The model under review builds one solid part; all positions refer to its coordinate system, in mm. A direction names the side the tool comes from. Round coordinates to 2 decimals unless told otherwise and drop trailing zeros. Loops run counter-clockwise (first coordinate to the right, second up) from the corner with the lowest first, then second, coordinate; pieces in that order, holes last. Notation, with made-up numbers: M 3,71 L 37,71 A27 cw 37,99 Z; hole C 3,-11 d10. An arc over 180 degrees is marked long. One line per question, with ' | ' between items.
from build123d import *

# Parameters (mm, degrees)
BOSS_EXTRUDE1_DEPTH = 5
SKETCH2_R           = 2.1
CUT_EXTRUDE1_DEPTH  = 10
SKETCH3_R           = 10
BOSS_EXTRUDE2_DEPTH = 1
SKETCH4_R           = 2.75
BOSS_EXTRUDE3_DEPTH = 5
SKETCH5_W           = 50
SKETCH5_H           = 30
SKETCH5_W_2         = 34
SKETCH5_H_2         = 14
CUT_EXTRUDE2_DEPTH  = 52.14684741
CUT_EXTRUDE3_START  = -1
CUT_EXTRUDE3_DEPTH  = 1
CUT_EXTRUDE4_START  = -1
CUT_EXTRUDE4_DEPTH  = 1
CHAMFER1_SIZE       = 3
CHAMFER2_SIZE       = 3
SKETCH8_W           = 10.980685111
SKETCH8_H           = 18.946061275
CUT_EXTRUDE5_DEPTH  = 51.645829048
BOSS_EXTRUDE4_DEPTH = 1


with BuildPart() as part:
    # Sketch1 → Boss-Extrude1 (new, symmetric)
    with BuildSketch(Plane.XY):
        Polygon((15, 5), (15, 0), (0, 0), (0, 19), (15, 19), (15, 14), (20, 14), (20, 24), (-10, 24), (-10, -5), (20, -5), (20, 5), align=None)
    extrude(amount=BOSS_EXTRUDE1_DEPTH, both=True)

    # Sketch2 → Cut-Extrude1 (cut)
    with BuildSketch(Plane.ZY.offset(10)):
        with Locations(Location((0, 9.5, 0), (0, 0, 270))):
            Circle(SKETCH2_R)
    extrude(amount=-CUT_EXTRUDE1_DEPTH, mode=Mode.SUBTRACT)

    # Sketch3 → Boss-Extrude2 (add)
    with BuildSketch(Plane(origin=(0, 24, 0), x_dir=(1, 0, 0), z_dir=(0, 1, 0))):
        with Locations(Location((0, 0, 0), (0, 0, 180))):
            Circle(SKETCH3_R)
    extrude(amount=BOSS_EXTRUDE2_DEPTH)

    # Sketch4 → Boss-Extrude3 (add)
    with BuildSketch(Plane(origin=(0, 0, 0), x_dir=(0.866025403784438, 0, 0.500000000000001), z_dir=(-0.500000000000001, 0, 0.866025403784438))):
        with BuildLine():
            Line((10, 25), (-10, 25))
            Line((-10, 25), (-4.615384615, 37.923076923))
            ThreePointArc((-4.615384615, 37.923076923), (0, 41), (4.615384615, 37.923076923))
            Line((4.615384615, 37.923076923), (10, 25))
        make_face()
        with Locations((0, 36)):
            Circle(SKETCH4_R, mode=Mode.SUBTRACT)
    extrude(amount=BOSS_EXTRUDE3_DEPTH)

    # Sketch5 → Cut-Extrude2 (cut, through all)
    with BuildSketch(Plane.XZ.offset(5)):
        with Locations((5, 0)):
            Rectangle(SKETCH5_W, SKETCH5_H)
        with Locations((5, 0)):
            Rectangle(SKETCH5_W_2, SKETCH5_H_2, mode=Mode.SUBTRACT)
    extrude(amount=-CUT_EXTRUDE2_DEPTH, mode=Mode.SUBTRACT)

    # Sketch6 → Cut-Extrude3 (cut)
    with BuildSketch(Plane(origin=(0, 25, 0), x_dir=(1, 0, 0), z_dir=(0, 1, 0)).offset(CUT_EXTRUDE3_START)):
        with BuildLine():
            Line((7.141428429, 7), (-7.141428429, 7))
            ThreePointArc((-7.141428429, 7), (-7.963874195, 6.047868038), (-8.660254038, 5))
            Line((-8.660254038, 5), (8.660254038, -5))
            ThreePointArc((8.660254038, -5), (9.920851384, 1.255670262), (7.141428429, 7))
        make_face()
    extrude(amount=CUT_EXTRUDE3_DEPTH, mode=Mode.SUBTRACT)

    # Sketch7 → Cut-Extrude4 (cut)
    with BuildSketch(Plane(origin=(0, 25, 0), x_dir=(1, 0, 0), z_dir=(0, 1, 0)).offset(CUT_EXTRUDE4_START)):
        with BuildLine():
            Line((-7.141428429, -7), (2.124355653, -7))
            Line((2.124355653, -7), (-10, 0))
            ThreePointArc((-10, 0), (-9.257815193, -3.780589618), (-7.141428429, -7))
        make_face()
    extrude(amount=CUT_EXTRUDE4_DEPTH, mode=Mode.SUBTRACT)

    # Chamfer1
    # the kernel refuses this chamfer: 3 mm, written as the material it adds along each edge
    with BuildSketch(Plane(origin=(5.341682432, 24, 8.857524482), x_dir=(0.013747938305293134, 0.9996219169112968, -0.023812127644090214), z_dir=(-0.8660254037844382, 0, -0.500000000000001))) as chamfer1_piece_1_section:
        Polygon((CHAMFER1_SIZE * 0.999621916911, -CHAMFER1_SIZE * 0.0274958766106), (-CHAMFER1_SIZE * 0.0274958766106, -CHAMFER1_SIZE * 0.999621916911), (0, 0), align=None)
    chamfer1_piece_1 = extrude(amount=25.430097928, mode=Mode.PRIVATE)
    chamfer1_piece_1 = split(chamfer1_piece_1, bisect_by=Plane(origin=(-10, 25.699033003, 2.85935222), z_dir=(1, 0, 0)), keep=Keep.TOP, mode=Mode.PRIVATE)
    chamfer1_piece_1 = split(chamfer1_piece_1, bisect_by=Plane(origin=(-6.251324666, 25.699033003, 5), z_dir=(0, 0, -1)), keep=Keep.TOP, mode=Mode.PRIVATE)
    add(chamfer1_piece_1)
    with BuildSketch(Plane(origin=(5.341682432, 24, 8.857524482), x_dir=(0.013747938305293134, 0.9996219169112968, -0.023812127644090214), z_dir=(-0.8660254037844382, 0, -0.500000000000001))) as chamfer1_piece_2_section:
        Polygon((CHAMFER1_SIZE * 0.999621916911, -CHAMFER1_SIZE * 0.0274958766106), (-CHAMFER1_SIZE * 0.0274958766106, -CHAMFER1_SIZE * 0.999621916911), (0, 0), align=None)
    chamfer1_piece_2 = extrude(amount=25.430097928, mode=Mode.PRIVATE)
    chamfer1_piece_2 = split(chamfer1_piece_2, bisect_by=Plane(origin=(-10.676225886, 25, 0.518721071), z_dir=(0, 1, 0)), keep=Keep.TOP, mode=Mode.PRIVATE)
    chamfer1_piece_2 = split(chamfer1_piece_2, bisect_by=Plane(origin=(-11.252418357, 25.835555068, 0.186056192), z_dir=(0.7994080650317889, -0.38461538461538497, 0.46153846153846245)), keep=Keep.TOP, mode=Mode.PRIVATE)
    chamfer1_piece_2 = split(chamfer1_piece_2, bisect_by=Plane(origin=(-10.676225886, 25.558334336, 5), z_dir=(0, 0, -1)), keep=Keep.TOP, mode=Mode.PRIVATE)
    add(chamfer1_piece_2)

    # Chamfer2
    # the kernel refuses this chamfer: 3 mm, written as the material it adds along each edge
    with BuildSketch(Plane(origin=(16.375303002, 24, 5), x_dir=(0, -0.9996219169112968, -0.02749587661058648), z_dir=(-1, 0, 0))) as chamfer2_piece_1_section:
        Polygon((CHAMFER2_SIZE * 0.999621916911, CHAMFER2_SIZE * 0.0274958766106), (-CHAMFER2_SIZE * 0.0274958766106, CHAMFER2_SIZE * 0.999621916911), (0, 0), align=None)
    chamfer2_piece_1 = extrude(amount=25.430097928, mode=Mode.PRIVATE)
    chamfer2_piece_1 = chamfer2_piece_1 & Plane(origin=(0, 22.869371877, 0), x_dir=(-1, 0, 0), z_dir=(0, -1, 0)) * Cylinder(10, 63, mode=Mode.PRIVATE)
    chamfer2_piece_1 = split(chamfer2_piece_1, bisect_by=Plane(origin=(4.051544609, 22.869371877, 7), z_dir=(0, 0, -1)), keep=Keep.TOP, mode=Mode.PRIVATE)
    chamfer2_piece_1 = split(chamfer2_piece_1, bisect_by=Plane(origin=(3.023607395, 22.869371877, 7.519183235), z_dir=(0.500000000000001, 0, -0.8660254037844382)), keep=Keep.TOP, mode=Mode.PRIVATE)
    add(chamfer2_piece_1)

    # Sketch8 → Cut-Extrude5 (cut, through all)
    with BuildSketch(Plane.XZ.offset(5)):
        with Locations((-15.490342555, -3.686972965)):
            Rectangle(SKETCH8_W, SKETCH8_H)
    extrude(amount=-CUT_EXTRUDE5_DEPTH, mode=Mode.SUBTRACT)

    # Sketch9 → Boss-Extrude4 (add)
    with BuildSketch(Plane(origin=(0, 24, 0), x_dir=(1, 0, 0), z_dir=(0, 1, 0))):
        with BuildLine():
            Line((-8.660254038, 5), (-10, 5))
            Line((-10, 5), (-10, 0))
            ThreePointArc((-10, 0), (-9.659258263, 2.588190451), (-8.660254038, 5))
        make_face()
    extrude(amount=BOSS_EXTRUDE4_DEPTH)


solid = part.part
1) Add section B-B on z = -3.75. State the section outline as (x, y) points, then the cut area to 3 significant figures.
Output values:
outline: M -10,-5 L 20,-5 L 20,5 L 15,5 L 15,0 L 0,0 L 0,19 L 15,19 L 15,14 L 20,14 L 20,24 L -6.5,24 L -6.5,31 L -9.38,25 L -10,25 Z | area: 552 mm²
2) Add section D-D on y = 19.5. State the section outline as (x, z) points.
Output values:
outline: M -10,-5 L 20,-5 L 20,5 L -10,5 Z
3) For line 1 (Z direction, x = -6.25, y = 9.5); line 2 (Y direction, x = 13, z = 1); line 3 (X direction, y = 4.5, z = 0.75), list the stretches that pass through material, from the lowest coordinate up.
Output values:
line 1: z = -5 to -2.1, 2.1 to 5 | line 2: y = -5 to 0, 19 to 24 | line 3: x = -10 to 0, 15 to 20
4) Insertion check: P1, Ø2, axis at x = 1.5, y = 25.5, coming from the -Z side; P2, Ø5, axis at x = 1, y = 32.5, coming from the -Z side; P3, Ø0.7, axis at x = -9, z = -4, coming from the +Y side; P4, Ø3, axis at y = 9.5, z = -0.5, coming from the +X side. Each pin has a flat end and moves straight along its axis. Give the tip position at first contact, or say it passes through.
Output values:
P1: stops at z = 0.29 | P2: stops at z = -0.87 | P3: stops at y = 26.33 | P4: passes through
5) Machinability: for faces 4 (the flat face through (4.82, 32.99, 4.99)), 5 (the flat face through (17, 14, 0)), 6 (the flat face through (-9.5, 25, -4.1)), 7 (the flat face through (15, 17, 0)), 8 (the flat face through (-2.506, 31.14, 4.327)), which of the approach directions +Z, -Z, +X, -X, +Y, -Y give a long, thin tool a straight path to every point of the face, cutting with its end or side? Answer none if there is none.
Output values:
face 4: +Z, +X, +Y | face 5: +Z, -Z, +X | face 6: -Z, -X, +Y | face 7: +Z, -Z | face 8: +Z, -X, +Y
6) Mouldability with a two-part tool opening along Y and no side actions: class faces 1 (the flat face through (-7.6, 31.4, -1.5)), 2 (the flat face through (-10, 11, -2)), 3 (the flat face through (15, 3, 0)) as +Y half, -Y half, draft (parallel to the pull), parting line (faces both ways), or undercut.
Output values:
face 1: +Y half | face 2: draft | face 3: undercut
7) Add section A-A on y = 8. State the section outline as (x, z) points.
Output values:
outline: M -10,-5 L 0,-5 L 0,-1.47 L -10,-1.47 Z; M -10,1.47 L 0,1.47 L 0,5 L -10,5 Z
8) Add section C-C on y = 34.5. State the section outline as (x, z) points, then the cut area to 3 significant figures.
Output values:
outline: M -7.73,1.31 L -5.23,-3.02 L -2,-1.15 L -4.5,3.18 Z; M -0.5,5.48 L 2,1.15 L 5.23,3.02 L 2.93,7 L 2.12,7 Z | area: 37.2 mm²
